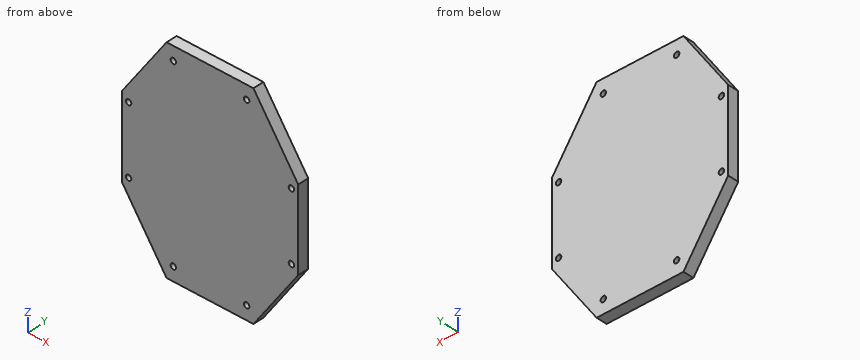
from build123d import *

# Parameters (mm, degrees)
SKETCH_1_R      = 2
EXTRUDE_1_DEPTH = 8


with BuildPart() as part:
    # 草图1 → 凸台-拉伸1 (new body)
    with BuildSketch(Plane(origin=(0, 0, 0), x_dir=(1, 0, 0), z_dir=(0, 1, 0))):
        Polygon((32, 53), (65, 5), (65, -55), (32, -103), (-32, -103), (-65, -55), (-65, 5), (-32, 53), align=None)
        with Locations((27, -93)):
            Circle(SKETCH_1_R, mode=Mode.SUBTRACT)
        with Locations((27, 43)):
            Circle(SKETCH_1_R, mode=Mode.SUBTRACT)
        with Locations((60, 0)):
            Circle(SKETCH_1_R, mode=Mode.SUBTRACT)
        with Locations((60, -50)):
            Circle(SKETCH_1_R, mode=Mode.SUBTRACT)
        with Locations((-27, -93)):
            Circle(SKETCH_1_R, mode=Mode.SUBTRACT)
        with Locations((-60, -50)):
            Circle(SKETCH_1_R, mode=Mode.SUBTRACT)
        with Locations((-60, 0)):
            Circle(SKETCH_1_R, mode=Mode.SUBTRACT)
        with Locations((-27, 43)):
            Circle(SKETCH_1_R, mode=Mode.SUBTRACT)
    extrude(amount=EXTRUDE_1_DEPTH)


solid = part.part
Source: CAD feature listing. Evaluate the final solid. Frame: model axes, mm. Give positions to 0.01 mm unless a question says otherwise; leave off trailing zeros. Order: outer loops, then holes, each group sorted by start corner. A loop starts at its lowest first (then second) coordinate and runs counter-clockwise, first axis right, second up. Notation, with made-up numbers: (5.5, -23) -> (43.5, -23) arc R13 ccw to (43.5, -11) -> close; hole circle Ø2 at (4, -2). An arc over 180 degrees is marked (long way). Use a Markdown table: item, result.
1) Ray query, line 1 along Z through (x, y) = (27, 2.5); line 2 along X through (y, z) = (6.25, 0); line 3 along X through (y, z) = (4, -43) (3 decimals). Return the intervals inside material, ascending. Write a range as [from, to].
Answer list:
| item | result |
|---|---|
| line 1 | [-53, -45], [-41, 91], [95, 103] |
| line 2 | [-65, -62], [-58, 58], [62, 65] |
| line 3 | [-38.875, -29], [-25, 25], [29, 38.875] |
2) Section query C-C, the plane y = 2.75. Count the separate pieces of the cut face and the enclosed holes in it, then the cut area to 3 significant figures.
Answer list:
| item | result |
|---|---|
| separate pieces | 1 |
| enclosed holes | 8 |
| area | 17,000 mm² |
3) Contact query for a flat-ended pin moving along its axis: P1, Ø1.5, axis at x = 49.5, y = 4.5, coming from the +Z side. Output: stop coordinate, or through.
Answer list:
| item | result |
|---|---|
| P1 | z = 78.64 |
4) Section query A-A, the plane x = 27. Return the cut outline in (y, z), then the cut area to 3 significant figures.
Answer list:
| item | result |
|---|---|
| outline | (0, -53) -> (8, -53) -> (8, -45) -> (0, -45) -> close; (0, -41) -> (8, -41) -> (8, 91) -> (0, 91) -> close; (0, 95) -> (8, 95) -> (8, 103) -> (0, 103) -> close |
| area | 1,180 mm² |
5) Section query D-D, the plane x = 43. Return the cut outline in (y, z), then the cut area to 3 significant figures.
Answer list:
| item | result |
|---|---|
| outline | (0, -37) -> (8, -37) -> (8, 87) -> (0, 87) -> close |
| area | 992 mm² |
6) Section query B-B, the plane z = 50. Return the cut outline in (x, y), then the cut area to 3 significant figures.
Answer list:
| item | result |
|---|---|
| outline | (-65, 0) -> (-62, 0) -> (-62, 8) -> (-65, 8) -> close; (-58, 0) -> (58, 0) -> (58, 8) -> (-58, 8) -> close; (62, 0) -> (65, 0) -> (65, 8) -> (62, 8) -> close |
| area | 976 mm² |
